Can you work these out from the model? Positions are in its coordinate system, mm. Face numbers are marked on the shaded views. Round coordinates to 2 decimals unless told otherwise and drop trailing zeros. Write each loop counter-clockwise with the first axis right and the second up, starting at its lowest first coordinate (ties: lowest second). Pieces come first, ordered by that corner, then holes. Notation, with made-up numbers: M -24,-6.75 L 32,-6.75 A8 cw 32,1.25 Z; hole C 55,-10.5 d7. An arc over 180 degrees is marked long. Use one line per item in the form item = value. Start each with the question number.
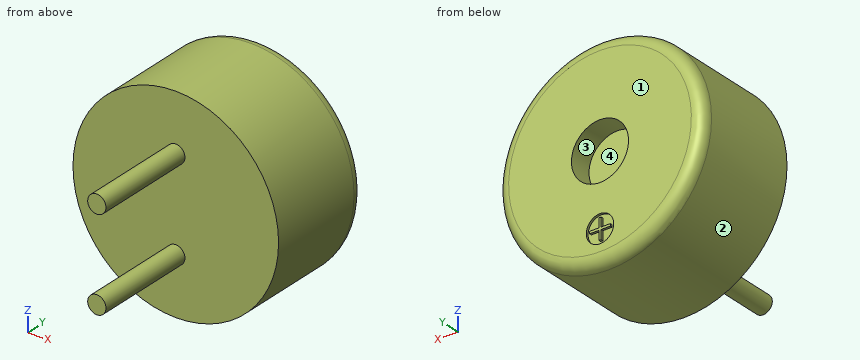
```python
from build123d import *

# Parameters (mm, degrees)
SKETCH1_R          = 4.5
EXTRUDE1_DEPTH     = 4.8
FILLET1_R          = 0.5
SKETCH6_R          = 0.4
EXTRUDE6_DEPTH     = 4.5
SKETCH2_R          = 1.25
CUT_EXTRUDE2_DEPTH = 1
SKETCH8_R          = 0.6
CUT_EXTRUDE3_DEPTH = 0.1


with BuildPart() as part:
    # Sketch1 → Extrude1 (new body)
    with BuildSketch(Plane(origin=(0, 0, 0), x_dir=(1, 0, 0), z_dir=(0, 1, 0))):
        with Locations(Location((0, 0, 0), (0, 0, 270))):
            Circle(SKETCH1_R)
    extrude(amount=EXTRUDE1_DEPTH)

    # Fillet1
    fillet1_edges = [part.edges().sort_by_distance(p)[0] for p in [
        (0, 4.8, -4.5),
    ]]
    fillet(fillet1_edges, radius=FILLET1_R)

    # Sketch6 → Extrude6 (add)
    with BuildSketch(Plane.XZ):
        with Locations(Location((0, -2, 0), (0, 0, 90))):
            Circle(SKETCH6_R)
        with Locations(Location((0, 2, 0), (0, 0, 90))):
            Circle(SKETCH6_R)
    extrude(amount=EXTRUDE6_DEPTH)

    # Sketch2 → Cut-Extrude2 (cut)
    with BuildSketch(Plane(origin=(0, 4.8, 0), x_dir=(1, 0, 0), z_dir=(0, 1, 0))):
        with Locations(Location((0, 0, 0), (0, 0, 270))):
            Circle(SKETCH2_R)
    extrude(amount=-CUT_EXTRUDE2_DEPTH, mode=Mode.SUBTRACT)

    # Sketch8 → Cut-Extrude3 (cut)
    with BuildSketch(Plane(origin=(0, 4.8, 0), x_dir=(1, 0, 0), z_dir=(0, 1, 0))):
        with Locations(Location((0, 3.083775569, 0), (0, 0, 270))):
            Circle(SKETCH8_R)
        Polygon((0.05, 3.533775569), (-0.05, 3.533775569), (-0.05, 3.133775569), (-0.45, 3.133775569), (-0.45, 3.033775569), (-0.05, 3.033775569), (-0.05, 2.633775569), (0.05, 2.633775569), (0.05, 3.033775569), (0.45, 3.033775569), (0.45, 3.133775569), (0.05, 3.133775569), align=None, mode=Mode.SUBTRACT)
    extrude(amount=-CUT_EXTRUDE3_DEPTH, mode=Mode.SUBTRACT)


solid = part.part
```
1. If we mould it in two halves opening along X, with no side actions, what happens to the marked faces 1, 2, 3 and 4? For each: pulls with the +X half, pulls with the -X half, needs draft (parallel to the pull), parting line crosses it, or undercut.
2. Will these pins go through, and if not, where does the flat tip stop? pin 1 (1 mm diameter, centred on x = -3, y = 3.5, fed in from +Z); pin 2 (1.5 mm diameter, centred on y = -2.5, z = -3.5, fed in from +X); pin 3 (4 mm diameter, centred on y = -1.5, z = 2.5, fed in from +X); pin 4 (0.8 mm diameter, centred on x = 0.5, z = 0, fed in from +Y).
3. If we section it at B-B (z = 0): List the corners of the cut face in (x, y) for me, and give its area (3 significant figures).
4. Please list where these lines run through material, in increasing order: line 1 along Y through (x, z) = (2, 1.25); line 2 along X through (y, z) = (4.4, 0); line 3 along X through (y, z) = (4.6, 0).
5. If we section it at A-A (y = -1.25): List the corners of the cut face in (x, z) for me.
6. If we section it at C-C (y = 2.75): List the corners of the cut face in (x, z) for me, and give its area (3 significant figures).
Model answer:
q1.face_1 = needs draft
q1.face_2 = parting line crosses it
q1.face_3 = undercut
q1.face_4 = undercut
q2.pin_1 = 3.74
q2.pin_2 = through
q2.pin_3 = 4.34
q2.pin_4 = 3.8
q3.outline = M -4.5,0 L 4.5,0 L 4.5,4.3 A0.5 ccw 4,4.8 L 1.25,4.8 L 1.25,3.8 L -1.25,3.8 L -1.25,4.8 L -4,4.8 A0.5 ccw -4.5,4.3 Z
q3.area = 40.6 mm2
q4.line_1 = 0 to 4.8
q4.line_2 = -4.49 to -1.25, 1.25 to 4.49
q4.line_3 = -4.4 to -1.25, 1.25 to 4.4
q5.outline = C 0,-2 d0.8; C 0,2 d0.8
q6.outline = C 0,0 d9
q6.area = 63.6 mm2
